Design review of the part built by this model. Coordinates are the model's own, in mm. A direction names the side the tool comes from. Coordinates: 2 decimals unless noted, no trailing zeros. Loops run counter-clockwise (first coordinate to the right, second up) from the corner with the lowest first, then second, coordinate; pieces in that order, holes last. Notation, with made-up numbers: (-31, 71) -> (-15, 71) arc R24 ccw to (-15, 81) -> close; hole circle Ø1 at (14.5, -27). An arc over 180 degrees is marked (long way). Use a Markdown table: item, result. Add a question column.
Q1. Take a section at D-D on z = -10.5. Write out the cut boundary in (x, y), plus the area to 3 significant figures.
Q2. For faces 1 (the face through (-30, -8, -12.5)), 2 (the face through (-52, 2, 0)), 3 (the face through (-4.256, -8.054, -1.788)), list the 3-axis set-ups (+Z, -Z, +X, -X, +Y, -Y) from which the entire face can be reached by the end or side of a thin tool; tool diameter is ignored.
Q3. Take a section at A-A on y = 0. Write out the cut boundary in (x, z) (3 decimals), plus the area to 3 significant figures.
Q4. Draft analysis for pull direction X (two halves, no side actions). For faces 4 (the face through (-4, 12.2, 0)), 5 (the face through (-8, 9, 0)), 6 (the face through (0, -8, 6)), 7 (the face through (-30, -7.8, 0)), state which applies: pulls with the +X half, pulls with the -X half, needs draft (parallel to the pull), parting line crosses it, or undercut.
Q5. For probe 1 along Z at (x, y) = (-3.25, 0); probe 2 along X at (y, z) = (9.75, -4.25); probe 3 along Y at (x, z) = (-30, 9.75), list the stretches that pass through material, from the lowest coordinate up.
Q6. Clearance check with flat-ended pins moving along their axes: pin 1 Ø5 at (x, z) = (-48, 10) entering from +Y; pin 2 Ø12 at (y, z) = (-2.5, 0) entering from +X (3 decimals); pin 3 Ø1 at (y, z) = (1.5, 4.5) entering from +X. State where each tip first meets the part, or that it passes through.
Q7. Take a section at C-C on x = -7. Write out the cut boundary in (y, z).
Q8. Take a section at B-B on z = 0. Write out the cut boundary in (x, y) (3 decimals), plus the area to 3 significant figures.
from build123d import *

# Parameters (mm, degrees)
SKETCH_1_W               = 60
SKETCH_1_H               = 28
EXTRUDE_1_DEPTH          = 12.5
CUT_EXTRUDE_1_DEPTH      = 64.292100613
CUT_EXTRUDE_1_DEPTH_BACK = 64.292100613
SKETCH_2_W               = 44
SKETCH_2_H               = 20
M18X1_51_D               = 16.5
M18X1_51_DEPTH           = 13
M18X1_51_CSINK_D         = 18.05
M18X1_51_CSINK_ANGLE     = 90
M18X1_51_TIP             = 4.957100107


with BuildPart() as part:
    # Эскиз1 → Бобышка-Вытянуть1 (new, symmetric)
    with BuildSketch(Plane.XY):
        with Locations((-30, -1.8)):
            Rectangle(SKETCH_1_W, SKETCH_1_H)
    extrude(amount=EXTRUDE_1_DEPTH, both=True)

    # Эскиз2 → Вырез-Вытянуть1 (cut, two sides: drawn at the far end of the back side and taken through both)
    with BuildSketch(Plane.XY.offset(-CUT_EXTRUDE_1_DEPTH_BACK)):
        with Locations((-30, 2.2)):
            Rectangle(SKETCH_2_W, SKETCH_2_H)
    extrude(amount=CUT_EXTRUDE_1_DEPTH + CUT_EXTRUDE_1_DEPTH_BACK, mode=Mode.SUBTRACT)

    # Отверстие обработанное метчиком M18x1.51
    with Locations(Plane(origin=(0, 0, 0), x_dir=(0, 0, -1), z_dir=(1, 0, 0))):
        with Locations((0, 0)):
            CounterSinkHole(M18X1_51_D / 2, M18X1_51_CSINK_D / 2, depth=M18X1_51_DEPTH, counter_sink_angle=M18X1_51_CSINK_ANGLE)
            with Locations((0, 0, -(M18X1_51_DEPTH + M18X1_51_TIP / 2))):  # 118° drill point
                Cone(0, M18X1_51_D / 2, M18X1_51_TIP, mode=Mode.SUBTRACT)


solid = part.part
Answer list:
| question | item | result |
|---|---|---|
| 1 | outline | (-60, -15.8) -> (0, -15.8) -> (0, 12.2) -> (-8, 12.2) -> (-8, -7.8) -> (-52, -7.8) -> (-52, 12.2) -> (-60, 12.2) -> close |
| 1 | area | 800 mm² |
| 2 | face 1 | -Z, +X, -X, +Y, -Y |
| 2 | face 2 | +Z, -Z, +Y |
| 2 | face 3 | +X |
| 3 | outline | (-60, -12.5) -> (-52, -12.5) -> (-52, 12.5) -> (-60, 12.5) -> close; (-8, -12.5) -> (0, -12.5) -> (0, -9.025) -> (-0.775, -8.25) -> (-8, -8.25) -> close; (-8, 8.25) -> (-0.775, 8.25) -> (0, 9.025) -> (0, 12.5) -> (-8, 12.5) -> close |
| 3 | area | 267 mm² |
| 4 | face 4 | needs draft |
| 4 | face 5 | undercut |
| 4 | face 6 | pulls with the +X half |
| 4 | face 7 | undercut |
| 5 | probe 1 | -12.5 to -8.25, 8.25 to 12.5 |
| 5 | probe 2 | -60 to -52, -8 to 0 |
| 5 | probe 3 | -15.8 to -7.8 |
| 6 | pin 1 | y = -7.8 |
| 6 | pin 2 | x = -0.525 |
| 6 | pin 3 | x = -52 |
| 7 | outline | (-15.8, -12.5) -> (12.2, -12.5) -> (12.2, 12.5) -> (-15.8, 12.5) -> close; hole circle Ø16.5 at (0, 0) |
| 8 | outline | (-60, -15.8) -> (0, -15.8) -> (0, -9.025) -> (-0.775, -8.25) -> (-13, -8.25) -> (-13.27, -7.8) -> (-52, -7.8) -> (-52, 12.2) -> (-60, 12.2) -> close; (-8, 8.25) -> (-0.775, 8.25) -> (0, 9.025) -> (0, 12.2) -> (-8, 12.2) -> close |
| 8 | area | 665 mm² |
